from build123d import *

# Parameters (mm, degrees)
SKETCH2_W           = 69.85
SKETCH2_H           = 6.35
BOSS_EXTRUDE1_DEPTH = 6.35
BOSS_EXTRUDE2_START = -12.7
SKETCH2_3_W         = 184.15
SKETCH2_3_H         = 44.45
SKETCH2_3_R         = 6.35
BOSS_EXTRUDE2_DEPTH = 12.7
SKETCH3_R           = 17.4625
CUT_EXTRUDE1_DEPTH  = 12.7


with BuildPart() as part:
    # Sketch2 → Boss-Extrude1 (new body)
    with BuildSketch(Plane(origin=(0, 0, 0), x_dir=(0, 0, -1), z_dir=(1, 0, 0))):
        with BuildLine():
            Line((-22.225, 22.225), (-22.225, 3.175))
            Line((-22.225, 3.175), (-5.499261314, 3.175))
            ThreePointArc((-5.499261314, 3.175), (0, 6.35), (5.499261314, 3.175))
            Line((5.499261314, 3.175), (22.225, 3.175))
            Line((22.225, 3.175), (22.225, 22.225))
            Line((22.225, 22.225), (-22.225, 22.225))
        make_face()
        with BuildLine():
            Line((-22.225, -3.175), (-22.225, -22.225))
            Line((-22.225, -22.225), (22.225, -22.225))
            Line((22.225, -22.225), (22.225, -3.175))
            Line((22.225, -3.175), (5.499261314, -3.175))
            ThreePointArc((5.499261314, -3.175), (0, -6.35), (-5.499261314, -3.175))
            Line((-5.499261314, -3.175), (-22.225, -3.175))
        make_face()
        with Locations((-57.15, 0)):
            Rectangle(SKETCH2_W, SKETCH2_H)
        with BuildLine():
            Line((5.499261314, -3.175), (22.225, -3.175))
            Line((22.225, -3.175), (22.225, 3.175))
            Line((22.225, 3.175), (5.499261314, 3.175))
            ThreePointArc((5.499261314, 3.175), (6.133628997, 1.643500936), (6.35, 0))
            ThreePointArc((6.35, 0), (6.133628997, -1.643500936), (5.499261314, -3.175))
        make_face()
        with BuildLine():
            Line((-22.225, 3.175), (-22.225, -3.175))
            Line((-22.225, -3.175), (-5.499261314, -3.175))
            ThreePointArc((-5.499261314, -3.175), (-6.35, 0), (-5.499261314, 3.175))
            Line((-5.499261314, 3.175), (-22.225, 3.175))
        make_face()
        with Locations((57.15, 0)):
            Rectangle(SKETCH2_W, SKETCH2_H)
    extrude(amount=BOSS_EXTRUDE1_DEPTH)

    # Sketch2_3 → Boss-Extrude2 (add)
    with BuildSketch(Plane(origin=(0, 0, 0), x_dir=(0, 0, -1), z_dir=(1, 0, 0)).offset(BOSS_EXTRUDE2_START)):
        Rectangle(SKETCH2_3_W, SKETCH2_3_H)
        Circle(SKETCH2_3_R, mode=Mode.SUBTRACT)
    extrude(amount=BOSS_EXTRUDE2_DEPTH)

    # Sketch3 → Cut-Extrude1 (cut)
    with BuildSketch(Plane.ZY.offset(12.7)):
        Circle(SKETCH3_R)
    extrude(amount=-CUT_EXTRUDE1_DEPTH, mode=Mode.SUBTRACT)


solid = part.part
Verification items for the finished model (mm, model axes). A direction names the side the tool comes from. Round coordinates to 2 decimals unless told otherwise and drop trailing zeros. Loops run counter-clockwise (first coordinate to the right, second up) from the corner with the lowest first, then second, coordinate; pieces in that order, holes last. Notation, with made-up numbers: M 53.5,70.25 L 105.5,70.25 A19 ccw 105.5,78.25 Z; hole C 38,53.25 d8. An arc over 180 degrees is marked long. Write each question's results on one line, items separated by ' | '.
1) Gauge pin test, flat ends, axial feed: P1, Ø15, axis at y = -12.5, z = 73.5, coming from the +X side; P2, Ø3, axis at x = 4, z = 70.5, coming from the -Y side (3 decimals); P3, Ø1.9, axis at x = 3, y = 9, coming from the +Z side (3 decimals); P4, Ø7, axis at x = 3, z = -71, coming from the +Y side (3 decimals). Record the tip position at first contact, or that the pin passes through.
Checks:
P1: stops at x = 0 | P2: stops at y = -3.175 | P3: stops at z = 22.225 | P4: stops at y = 22.225
2) Section check B-B on x = -4.5. Record the boundary of the cut face in (y, z) (1 decimal), then the cut area to 3 significant figures.
Checks:
outline: M -22.2,-92.1 L 22.2,-92.1 L 22.2,92.1 L -22.2,92.1 Z; hole C 0,0 d34.9 | area: 7,230 mm2
3) Scan lines: L1, parallel to Y at x = -9.25, z = 0 (1 decimal); L2, parallel to X at y = -6.5, z = 2; L3, parallel to X at y = -13, z = -25. Record each from-to range of solid material in increasing order. Write a range as from..to.
Checks:
L1: y = -22.2..-17.5, 17.5..22.2 | L2: x = 0..6.35 | L3: x = -12.7..0
4) Mould release check, pull along Z, two halves, no side actions. Record for faces 1 (the flat face through (-5, -22.225, 1)), 2 (the flat face through (0, 0, 8)), 3 (the flat face through (-5, 0, -92.075)): released by +Z, released by -Z, zero draft, split by the parting line, or undercut.
Checks:
face 1: zero draft | face 2: undercut | face 3: released by -Z
5) Section check D-D on y = 9. Record the boundary of the cut face in (x, z) (3 decimals).
Checks:
outline: M -12.7,-92.075 L 0,-92.075 L 0,-22.225 L 6.35,-22.225 L 6.35,22.225 L 0,22.225 L 0,92.075 L -12.7,92.075 L -12.7,14.965 L 0,14.965 L 0,-14.965 L -12.7,-14.965 Z
6) Section check C-C on z = 60.5. Record the boundary of the cut face in (x, y) (3 decimals), then the cut area to 3 significant figures.
Checks:
outline: M -12.7,-22.225 L 0,-22.225 L 0,-3.175 L 6.35,-3.175 L 6.35,3.175 L 0,3.175 L 0,22.225 L -12.7,22.225 Z | area: 605 mm2
7) Access from +Z, -Z, +X, -X, +Y, -Y to the whole of each face (thin tool, end or side, straight path). Record for faces 4 (the cylindrical face through (-6.439, -10.626, -13.858)), 5 (the flat face through (3, -13, 22.225)), 6 (the flat face through (0, 13, 58)), 7 (the flat face through (0, 13, -57)).
Checks:
face 4: -X | face 5: +Z, +X, -Y | face 6: +Z, +X, +Y | face 7: -Z, +X, +Y
